```python
from build123d import *

# Parameters (mm, degrees)
SKETCH1_W                = 13
SKETCH1_H                = 50
SKETCH1_R                = 3.175
BOSS_EXTRUDE1_DEPTH      = 76.2
SKETCH2_W                = 13
SKETCH2_H                = 25
CUT_EXTRUDE1_DEPTH       = 10
M4_CLEARANCE_HOLE1_D     = 4.3
M4_CLEARANCE_HOLE1_DEPTH = 5
M4_CLEARANCE_HOLE1_TIP   = 1.291850331
M4_CLEARANCE_HOLE2_D     = 4.3
M4_CLEARANCE_HOLE2_DEPTH = 5
M4_CLEARANCE_HOLE2_TIP   = 1.291850331
FILLET1_R                = 3


with BuildPart() as part:
    # Sketch1 → Boss-Extrude1 (new body)
    with BuildSketch(Plane.XY):
        with Locations((6.5, 25)):
            Rectangle(SKETCH1_W, SKETCH1_H)
        with Locations((6.5, 45)):
            Circle(SKETCH1_R, mode=Mode.SUBTRACT)
    extrude(amount=BOSS_EXTRUDE1_DEPTH)

    # Sketch2 → Cut-Extrude1 (cut, symmetric)
    with BuildSketch(Plane.XY.offset(62.55)):
        with Locations((6.5, 37.5)):
            Rectangle(SKETCH2_W, SKETCH2_H)
    extrude(amount=CUT_EXTRUDE1_DEPTH, both=True, mode=Mode.SUBTRACT)

    # M4 Clearance Hole1
    with Locations(Plane(origin=(0, 0, 0), x_dir=(-1, 0, 0), z_dir=(0, 0, -1))):
        with Locations((-6.579246302, 18), (-6.579246302, 6)):
            Hole(M4_CLEARANCE_HOLE1_D / 2, depth=M4_CLEARANCE_HOLE1_DEPTH)
            with Locations((0, 0, -(M4_CLEARANCE_HOLE1_DEPTH + M4_CLEARANCE_HOLE1_TIP / 2))):  # 118° drill point
                Cone(0, M4_CLEARANCE_HOLE1_D / 2, M4_CLEARANCE_HOLE1_TIP, mode=Mode.SUBTRACT)

    # M4 Clearance Hole2
    with Locations(Plane.XY.offset(76.2)):
        with Locations((6.579246302, 18), (6.579246302, 6)):
            Hole(M4_CLEARANCE_HOLE2_D / 2, depth=M4_CLEARANCE_HOLE2_DEPTH)
            with Locations((0, 0, -(M4_CLEARANCE_HOLE2_DEPTH + M4_CLEARANCE_HOLE2_TIP / 2))):  # 118° drill point
                Cone(0, M4_CLEARANCE_HOLE2_D / 2, M4_CLEARANCE_HOLE2_TIP, mode=Mode.SUBTRACT)

    # Fillet1
    fillet1_edges = [part.edges().sort_by_distance(p)[0] for p in [
        (0, 50, 26.275),
        (13, 50, 26.275),
        (0, 50, 74.375),
        (13, 50, 74.375),
        (13, 0, 38.1),
        (0, 0, 38.1),
    ]]
    fillet(fillet1_edges, radius=FILLET1_R)


solid = part.part
```
Verification items for the finished model (mm, model axes). A direction names the side the tool comes from. Give positions to 0.01 mm unless a question says otherwise; leave off trailing zeros. Loops run counter-clockwise (first coordinate to the right, second up) from the corner with the lowest first, then second, coordinate; pieces in that order, holes last.
1. Section check B-B, the plane z = 46. Enter the section's corners in (x, y) (3 decimals).
2. Thickness scan on line 1 (Y direction, x = 6.5, z = 74.6) (3 decimals); line 2 (Z direction, x = 9.5, y = 43.5); line 3 (X direction, y = 45, z = 73.45) (3 decimals). Record the ranges inside material, lowest first.
3. Mould release check, pull along X, two halves, no side actions. Record for faces 5 (the flat face through (6, 38, 72.55)), 6 (the cylindrical face through (4.53, 6.65, 73.67)), 7 (the cylindrical face through (12.1, 49.14, 26.64)): released by +X, released by -X, zero draft, split by the parting line, or undercut.
4. Go/stop test with flat-tipped pins: pin 1 Ø4 at (x, y) = (6.58, 6) entering from +Z; pin 2 Ø3.5 at (x, y) = (6.58, 18) entering from +Z; pin 3 Ø5.5 at (x, y) = (6.5, 45) entering from +Z. Record where each tip stops, or that it passes through.
5. Section check D-D, the plane z = 55.5. Enter the section's corners in (x, y).
6. Set-up check for faces 1 (the flat face through (6, 25, 0)), 2 (the cylindrical face through (6.11, 15.9, 2.54)), 3 (the cylindrical face through (5.59, 16.09, 73.67)), 4 (the flat face through (6, 38, 52.55)): record each of +Z, -Z, +X, -X, +Y, -Y from which the full face is reachable in a straight line by a thin tool's end or side.
7. Section check C-C, the plane x = 11.75. Enter the section's corners in (y, z).
8. Section check A-A, the plane y = 45. Enter the section's corners in (x, z) (3 decimals).
Geometry says:
1. outline: (0, 3) arc R3 ccw to (3, 0) - (10, 0) arc R3 ccw to (13, 3) - (13, 47) arc R3 ccw to (10, 50) - (3, 50) arc R3 ccw to (0, 47) - close; hole circle Ø6.35 at (6.5, 45)
2. line 1: y = 0 to 3.851, 8.149 to 15.851, 20.149 to 41.825, 48.175 to 50
2. line 2: z = 0 to 52.55, 72.55 to 76.2
2. line 3: x = 0 to 3.325, 9.675 to 13
3. face 5: zero draft
3. face 6: undercut
3. face 7: released by +X
4. pin 1: stops at z = 71.11
4. pin 2: stops at z = 70.96
4. pin 3: passes through
5. outline: (0, 3) arc R3 ccw to (3, 0) - (10, 0) arc R3 ccw to (13, 3) - (13, 25) - (0, 25) - close
6. face 1: -Z, +X, -X, +Y, -Y
6. face 2: -Z
6. face 3: +Z
6. face 4: +X, -X, +Y
7. outline: (0.56, 0) - (49.44, 0) - (49.44, 52.55) - (25, 52.55) - (25, 72.55) - (49.44, 72.55) - (49.44, 76.2) - (0.56, 76.2) - close
8. outline: (0, 0) - (3.325, 0) - (3.325, 52.55) - (0, 52.55) - close; (0, 72.55) - (3.325, 72.55) - (3.325, 76.2) - (0, 76.2) - close; (9.675, 0) - (13, 0) - (13, 52.55) - (9.675, 52.55) - close; (9.675, 72.55) - (13, 72.55) - (13, 76.2) - (9.675, 76.2) - close
